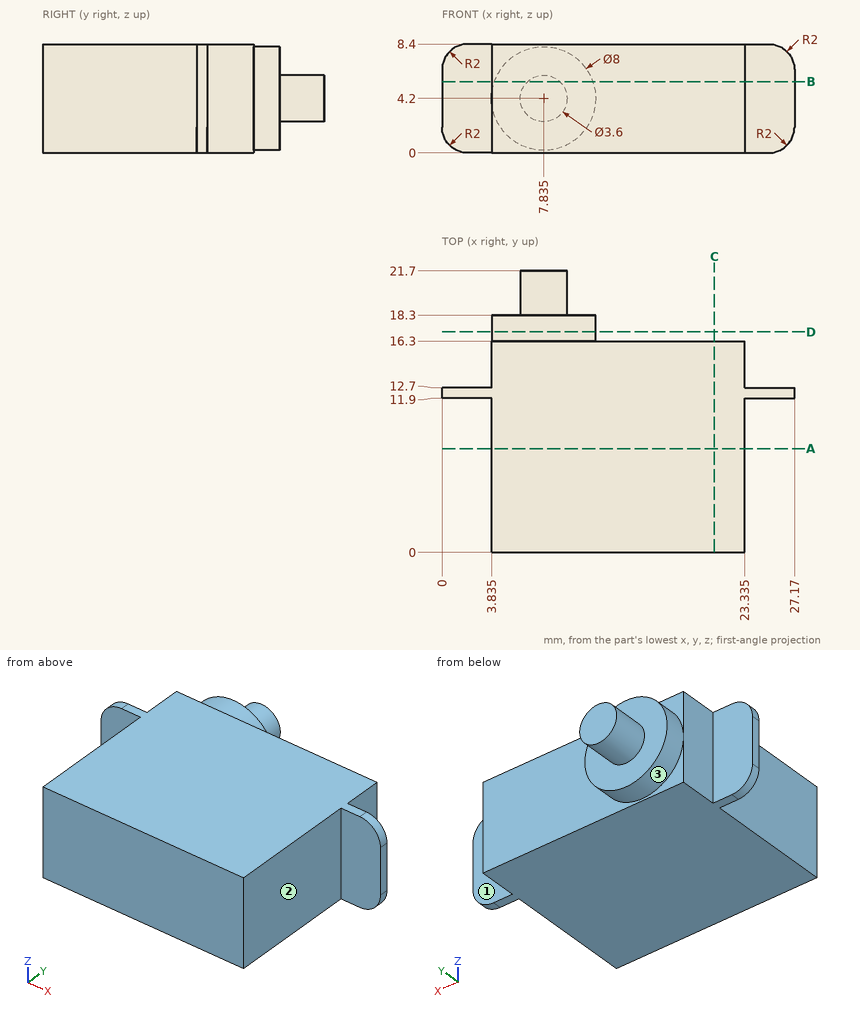
Print and shaded views of the part. All mm, measured from the part's lowest x, y and z. A direction names the side the tool comes from. Round coordinates to 2 decimals unless told otherwise and drop trailing zeros. Write each loop counter-clockwise with the first axis right and the second up, starting at its lowest first coordinate (ties: lowest second). Pieces come first, ordered by that corner, then holes.
(1) 3-axis set-ups, long thin cutter, end or side, ignore diameter. For the marked faces 1, 2 and 3: which of +Z, -Z, +X, -X, +Y, -Y reach the whole face in a straight line?
(2) Slice it at D-D, the plane y = 17. Write the cut outline in (x, z) (3 decimals).
(3) Slice it at A-A, the plane y = 8. Write the cut outline in (x, z) (3 decimals).
(4) Slice it at B-B, the plane z = 5.5. Write the cut outline in (x, y) (3 decimals).
(5) Slice it at C-C, the plane x = 21. Write the cut outline in (y, z), and give its area (3 significant figures).
(6) Drop flat-ended pins along their axis: P1, Ø4, axis at x = 25.5, z = 5, coming from the -Y side; P2, Ø4, axis at y = 8, z = 2.5, coming from the -X side (3 decimals); P3, Ø2.5, axis at y = 6, z = 5, coming from the +X side (3 decimals). Give the stop position or say it passes through.
(7) Probe line 1 along Y through (x, z) = (23.75, 3); line 2 along Y through (x, z) = (5, 5); line 3 along X through (y, z) = (13, 0.75) (3 decimals). List the from-to ranges inside material, lowest first.
From the geometry:
1. face 1: +Z, -Z, +X, +Y
1. face 2: +Z, -Z, +X, -Y
1. face 3: +Y
2. outline: circle Ø8 at (7.835, 4.2)
3. outline: (3.835, 0) - (23.335, 0) - (23.335, 8.4) - (3.835, 8.4) - close
4. outline: (0, 11.9) - (3.835, 11.9) - (3.835, 0) - (23.335, 0) - (23.335, 11.9) - (27.17, 11.9) - (27.17, 12.7) - (23.335, 12.7) - (23.335, 16.3) - (11.618, 16.3) - (11.618, 18.3) - (9.08, 18.3) - (9.08, 21.7) - (6.59, 21.7) - (6.59, 18.3) - (4.052, 18.3) - (4.052, 16.3) - (3.835, 16.3) - (3.835, 12.7) - (0, 12.7) - close
5. outline: (0, 0) - (16.3, 0) - (16.3, 8.4) - (0, 8.4) - close
5. area: 137 mm2
6. P1: stops at y = 11.9
6. P2: stops at x = 3.835
6. P3: stops at x = 23.335
7. line 1: y = 11.9 to 12.7
7. line 2: y = 0 to 18.3
7. line 3: x = 3.835 to 23.335
